Geometry check sheet. Reference: the model listing, model coordinates, mm. Round coordinates to 2 decimals unless told otherwise and drop trailing zeros.
(1) Gauge pin test, flat ends, axial feed: P1, Ø5, axis at x = 4.5, y = 4, coming from the -Z side; P2, Ø2, axis at x = 1.5, z = 296.5, coming from the -Y side; P3, Ø1.4, axis at y = 1.5, z = 179.5, coming from the +X side; P4, Ø2, axis at x = 1.5, z = 244.5, coming from the +Y side. Record the tip position at first contact, or that the pin passes through.
(2) Thickness scan on L1, parallel to Y at x = -7.25, z = 122.5; L2, parallel to Y at x = -0.5, z = 216; L3, parallel to Y at x = -4.5, z = 192. Record the ranges inside material, lowest first.
(3) Cross-section at A-A on z = 306. Count the separate pieces of the cut face and the enclosed holes in it, and give its area (3 significant figures).
from build123d import *

# Parameters (mm, degrees)
SKETCH1_R           = 2.1
BOSS_EXTRUDE2_DEPTH = 500


with BuildPart() as part:
    # Sketch1 → Boss-Extrude2 (new body)
    with BuildSketch(Plane.XY):
        with BuildLine():
            Line((-8.5, 10), (-4.862792737, 10))
            ThreePointArc((-4.862792737, 10), (-4.598292737, 9.947387679), (-4.374060464, 9.797560464))
            Line((-4.374060464, 9.797560464), (-3.3865, 8.81))
            Line((-3.3865, 8.81), (-3.3865, 8.2))
            Line((-3.3865, 8.2), (-5.5, 8.2))
            Line((-5.5, 8.2), (-5.5, 6.561))
            Line((-5.5, 6.561), (-2.8395, 3.9005))
            Line((-2.8395, 3.9005), (-0.1, 3.9005))
            Line((-0.1, 3.9005), (0, 3.8005))
            Line((0, 3.8005), (0.1, 3.9005))
            Line((0.1, 3.9005), (2.8395, 3.9005))
            Line((2.8395, 3.9005), (5.5, 6.561))
            Line((5.5, 6.561), (5.5, 8.2))
            Line((5.5, 8.2), (3.3865, 8.2))
            Line((3.3865, 8.2), (3.3865, 8.81))
            Line((3.3865, 8.81), (4.374060464, 9.797560464))
            ThreePointArc((4.374060464, 9.797560464), (4.598292737, 9.947387679), (4.862792737, 10))
            Line((4.862792737, 10), (8.5, 10))
            ThreePointArc((8.5, 10), (9.560660172, 9.560660172), (10, 8.5))
            Line((10, 8.5), (10, 4.862792737))
            ThreePointArc((10, 4.862792737), (9.947387679, 4.598292737), (9.797560464, 4.374060464))
            Line((9.797560464, 4.374060464), (8.81, 3.3865))
            Line((8.81, 3.3865), (8.2, 3.3865))
            Line((8.2, 3.3865), (8.2, 5.5))
            Line((8.2, 5.5), (6.561, 5.5))
            Line((6.561, 5.5), (3.9005, 2.8395))
            Line((3.9005, 2.8395), (3.9005, 0.1))
            Line((3.9005, 0.1), (3.8005, 0))
            Line((3.8005, 0), (3.9005, -0.1))
            Line((3.9005, -0.1), (3.9005, -2.8395))
            Line((3.9005, -2.8395), (6.561, -5.5))
            Line((6.561, -5.5), (8.2, -5.5))
            Line((8.2, -5.5), (8.2, -3.3865))
            Line((8.2, -3.3865), (8.81, -3.3865))
            Line((8.81, -3.3865), (9.797560464, -4.374060464))
            ThreePointArc((9.797560464, -4.374060464), (9.947387679, -4.598292737), (10, -4.862792737))
            Line((10, -4.862792737), (10, -15.137207263))
            ThreePointArc((10, -15.137207263), (9.947387679, -15.401707263), (9.797560464, -15.625939536))
            Line((9.797560464, -15.625939536), (8.81, -16.6135))
            Line((8.81, -16.6135), (8.2, -16.6135))
            Line((8.2, -16.6135), (8.2, -14.5))
            Line((8.2, -14.5), (6.561, -14.5))
            Line((6.561, -14.5), (3.9005, -17.1605))
            Line((3.9005, -17.1605), (3.9005, -19.9))
            Line((3.9005, -19.9), (3.8005, -20))
            Line((3.8005, -20), (3.9005, -20.1))
            Line((3.9005, -20.1), (3.9005, -22.8395))
            Line((3.9005, -22.8395), (6.561, -25.5))
            Line((6.561, -25.5), (8.2, -25.5))
            Line((8.2, -25.5), (8.2, -23.3865))
            Line((8.2, -23.3865), (8.81, -23.3865))
            Line((8.81, -23.3865), (9.797560464, -24.374060464))
            ThreePointArc((9.797560464, -24.374060464), (9.947387679, -24.598292737), (10, -24.862792737))
            Line((10, -24.862792737), (10, -28.5))
            ThreePointArc((10, -28.5), (9.560660172, -29.560660172), (8.5, -30))
            Line((8.5, -30), (4.862792737, -30))
            ThreePointArc((4.862792737, -30), (4.598292737, -29.947387679), (4.374060464, -29.797560464))
            Line((4.374060464, -29.797560464), (3.3865, -28.81))
            Line((3.3865, -28.81), (3.3865, -28.2))
            Line((3.3865, -28.2), (5.5, -28.2))
            Line((5.5, -28.2), (5.5, -26.561))
            Line((5.5, -26.561), (2.8395, -23.9005))
            Line((2.8395, -23.9005), (0.1, -23.9005))
            Line((0.1, -23.9005), (0, -23.8005))
            Line((0, -23.8005), (-0.1, -23.9005))
            Line((-0.1, -23.9005), (-2.8395, -23.9005))
            Line((-2.8395, -23.9005), (-5.5, -26.561))
            Line((-5.5, -26.561), (-5.5, -28.2))
            Line((-5.5, -28.2), (-3.3865, -28.2))
            Line((-3.3865, -28.2), (-3.3865, -28.81))
            Line((-3.3865, -28.81), (-4.374060464, -29.797560464))
            ThreePointArc((-4.374060464, -29.797560464), (-4.598292737, -29.947387679), (-4.862792737, -30))
            Line((-4.862792737, -30), (-8.5, -30))
            ThreePointArc((-8.5, -30), (-9.560660172, -29.560660172), (-10, -28.5))
            Line((-10, -28.5), (-10, -24.862792737))
            ThreePointArc((-10, -24.862792737), (-9.947387679, -24.598292737), (-9.797560464, -24.374060464))
            Line((-9.797560464, -24.374060464), (-8.81, -23.3865))
            Line((-8.81, -23.3865), (-8.2, -23.3865))
            Line((-8.2, -23.3865), (-8.2, -25.5))
            Line((-8.2, -25.5), (-6.561, -25.5))
            Line((-6.561, -25.5), (-3.9005, -22.8395))
            Line((-3.9005, -22.8395), (-3.9005, -20.1))
            Line((-3.9005, -20.1), (-3.8005, -20))
            Line((-3.8005, -20), (-3.9005, -19.9))
            Line((-3.9005, -19.9), (-3.9005, -17.1605))
            Line((-3.9005, -17.1605), (-6.561, -14.5))
            Line((-6.561, -14.5), (-8.2, -14.5))
            Line((-8.2, -14.5), (-8.2, -16.6135))
            Line((-8.2, -16.6135), (-8.81, -16.6135))
            Line((-8.81, -16.6135), (-9.797560464, -15.625939536))
            ThreePointArc((-9.797560464, -15.625939536), (-9.947387679, -15.401707263), (-10, -15.137207263))
            Line((-10, -15.137207263), (-10, -4.862792737))
            ThreePointArc((-10, -4.862792737), (-9.947387679, -4.598292737), (-9.797560464, -4.374060464))
            Line((-9.797560464, -4.374060464), (-8.81, -3.3865))
            Line((-8.81, -3.3865), (-8.2, -3.3865))
            Line((-8.2, -3.3865), (-8.2, -5.5))
            Line((-8.2, -5.5), (-6.561, -5.5))
            Line((-6.561, -5.5), (-3.9005, -2.8395))
            Line((-3.9005, -2.8395), (-3.9005, -0.1))
            Line((-3.9005, -0.1), (-3.8005, 0))
            Line((-3.8005, 0), (-3.9005, 0.1))
            Line((-3.9005, 0.1), (-3.9005, 2.8395))
            Line((-3.9005, 2.8395), (-6.561, 5.5))
            Line((-6.561, 5.5), (-8.2, 5.5))
            Line((-8.2, 5.5), (-8.2, 3.3865))
            Line((-8.2, 3.3865), (-8.81, 3.3865))
            Line((-8.81, 3.3865), (-9.797560464, 4.374060464))
            ThreePointArc((-9.797560464, 4.374060464), (-9.947387679, 4.598292737), (-10, 4.862792737))
            Line((-10, 4.862792737), (-10, 8.5))
            ThreePointArc((-10, 8.5), (-9.560660172, 9.560660172), (-8.5, 10))
        make_face()
        Circle(SKETCH1_R, mode=Mode.SUBTRACT)
        with Locations((0, -20)):
            Circle(SKETCH1_R, mode=Mode.SUBTRACT)
        Polygon((-8.2, -12.7), (-8.2, -7.3), (-6.239, -7.3), (-5.5, -6.561), (-2.8395, -3.9005), (-0.1, -3.9005), (0, -3.8005), (0.1, -3.9005), (2.8395, -3.9005), (5.5, -6.561), (6.239, -7.3), (8.2, -7.3), (8.2, -12.7), (6.239, -12.7), (5.5, -13.439), (2.8395, -16.0995), (0.1, -16.0995), (0, -16.1995), (-0.1, -16.0995), (-2.8395, -16.0995), (-5.5, -13.439), (-6.239, -12.7), align=None, mode=Mode.SUBTRACT)
    extrude(amount=BOSS_EXTRUDE2_DEPTH)


solid = part.part
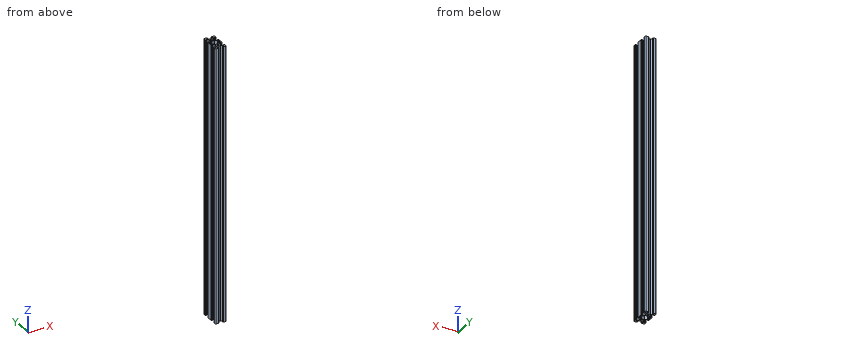
Found:
1. P1: stops at z = 0
1. P2: stops at y = -23.9
1. P3: stops at x = 3.9
1. P4: stops at y = 3.9
2. L1: y = -30 to -25.5, -14.5 to -12.7, -7.3 to -5.5, 5.5 to 10
2. L2: y = -23.9 to -22.04, -17.96 to -16.1, -3.9 to -2.04, 2.04 to 3.9
2. L3: y = -29.9 to -28.2, -25.56 to -23.44, -16.56 to -14.44, -5.56 to -3.44, 3.44 to 5.56, 8.2 to 9.9
3. separate pieces: 1
3. enclosed holes: 3
3. area: 297 mm2
